Could you check a few things on this model? Use its own coordinates, in mm. Give positions to 0.01 mm unless a question says otherwise; leave off trailing zeros. Order: outer loops, then holes, each group sorted by start corner. A loop starts at its lowest first (then second) coordinate and runs counter-clockwise, first axis right, second up.
from build123d import *

# Parameters (mm, degrees)
SKETCH_R        = 50
PAD_DEPTH       = 32
SKETCH001_R     = 48
POCKET_DEPTH    = 30
SKETCH002_R     = 4
PAD001_DEPTH    = 30
SKETCH005_W     = 9.3
SKETCH005_H     = 11.3
POCKET001_DEPTH = 10
SKETCH006_W     = 6
SKETCH006_H     = 9
PAD004_DEPTH    = 10
POCKET002_DEPTH = 8
SKETCH009_R     = 5
PAD006_DEPTH    = 4
SKETCH011_W     = 0.5
SKETCH011_H     = 9.3
PAD007_DEPTH    = 0.5
SKETCH012_R     = 5
PAD008_DEPTH    = 3
POCKET004_DEPTH = 2
SKETCH014_R     = 1.5
POCKET005_DEPTH = 4
POCKET006_DEPTH = 2
SKETCH015_R     = 1.5
POCKET007_DEPTH = 5
SKETCH016_R     = 2
POCKET008_DEPTH = 5.8


with BuildPart() as part:
    # Sketch → Pad (new body)
    with BuildSketch(Plane.XY):
        Circle(SKETCH_R)
    extrude(amount=PAD_DEPTH)

    # Sketch001 (on DatumPlane) → Pocket (cut)
    with BuildSketch(Plane.XY.offset(32)):
        Circle(SKETCH001_R)
    extrude(amount=-POCKET_DEPTH, mode=Mode.SUBTRACT)

    # Sketch002 (on DatumPlane) → Pad001 (join)
    with BuildSketch(Plane.XY.offset(32)):
        with Locations((-36.373067, 21)):
            Circle(SKETCH002_R)
        with Locations((0, -42)):
            Circle(SKETCH002_R)
        with Locations((36.373067, 21)):
            Circle(SKETCH002_R)
    extrude(amount=-PAD001_DEPTH)

    # Sketch005 (on DatumPlane) → Pocket001 (cut)
    with BuildSketch(Plane.YZ.offset(50)):
        with Locations((0, 7.65)):
            Rectangle(SKETCH005_W, SKETCH005_H)
    extrude(amount=-POCKET001_DEPTH, mode=Mode.SUBTRACT)

    # Sketch006 (on DatumPlane) → Pad004 (join)
    with BuildSketch(Plane.XY.offset(2)):
        with Locations((40, 0)):
            Rectangle(SKETCH006_W, SKETCH006_H)
    extrude(amount=PAD004_DEPTH)

    # Sketch007 (on Face14 of Pad004) → Pocket002 (cut)
    with BuildSketch(Plane(origin=(37, 0, 0), x_dir=(0, -1, 0), z_dir=(-1, 0, 0))):
        with BuildLine():
            ThreePointArc((-3.99875, 6.6), (0, 2.7), (3.99875, 6.6))
            Line((5.575286, 6.6), (3.99875, 6.6))
            Line((5.575286, 15.969053), (5.575286, 6.6))
            Line((-6.906295, 15.969053), (5.575286, 15.969053))
            Line((-6.906295, 6.6), (-6.906295, 15.969053))
            Line((-3.99875, 6.6), (-6.906295, 6.6))
        make_face()
    extrude(amount=-POCKET002_DEPTH, mode=Mode.SUBTRACT)

    # Sketch009 (on DatumPlane) → Pad006 (join)
    with BuildSketch(Plane.XY.offset(2)):
        with Locations((-22.75, 32.75)):
            Circle(SKETCH009_R)
        with Locations((22.75, 32.75)):
            Circle(SKETCH009_R)
        with Locations((22.75, -32.75)):
            Circle(SKETCH009_R)
        with Locations((-22.75, -32.75)):
            Circle(SKETCH009_R)
    extrude(amount=PAD006_DEPTH)

    # Sketch011 (on DatumPlane) → Pad007 (join)
    with BuildSketch(Plane.XY.offset(2)):
        with Locations((49.533305, 0)):
            Rectangle(SKETCH011_W, SKETCH011_H)
    extrude(amount=PAD007_DEPTH)

    # Sketch012 (on DatumPlane) → Pad008 (join)
    with BuildSketch(Plane.XY.offset(2)):
        with Locations((37.35, -11.5)):
            Circle(SKETCH012_R)
    pad008 = extrude(amount=PAD008_DEPTH)

    # Sketch013 (on Face33 of Pad008) → Pocket004 (cut)
    with BuildSketch(Plane.XY.offset(5)):
        Polygon((39.95, -13.001111), (39.95, -9.998889), (37.35, -8.497779), (34.75, -9.998889), (34.75, -13.001111), (37.35, -14.502221), align=None)
    pocket004 = extrude(amount=-POCKET004_DEPTH, mode=Mode.SUBTRACT)

    # Sketch014 (on Face33 of Pocket004) → Pocket005 (cut)
    with BuildSketch(Plane.XY.offset(5)):
        with Locations((37.35, -11.5)):
            Circle(SKETCH014_R)
    pocket005 = extrude(amount=-POCKET005_DEPTH, mode=Mode.SUBTRACT)

    # Sketch010 (on DatumPlane) → Pocket006 (cut)
    with BuildSketch(Plane.XY.offset(6)):
        Polygon((-20.15, 31.248889), (-20.15, 34.251111), (-22.75, 35.752221), (-25.35, 34.251111), (-25.35, 31.248889), (-22.75, 29.747779), align=None)
        Polygon((25.35, -34.251111), (25.35, -31.248889), (22.75, -29.747779), (20.15, -31.248889), (20.15, -34.251111), (22.75, -35.752221), align=None)
        Polygon((22.75, 35.752221), (20.15, 34.251111), (20.15, 31.248889), (22.75, 29.747779), (25.35, 31.248889), (25.35, 34.251111), align=None)
        Polygon((-20.15, -31.248889), (-22.75, -29.747779), (-25.35, -31.248889), (-25.35, -34.251111), (-22.75, -35.752221), (-20.15, -34.251111), align=None)
    extrude(amount=-POCKET006_DEPTH, mode=Mode.SUBTRACT)

    # Sketch015 (on DatumPlane) → Pocket007 (cut)
    with BuildSketch(Plane.XY.offset(6)):
        with Locations((-22.75, 32.75)):
            Circle(SKETCH015_R)
        with Locations((22.75, 32.75)):
            Circle(SKETCH015_R)
        with Locations((22.7, -32.75)):
            Circle(SKETCH015_R)
        with Locations((-22.75, -32.75)):
            Circle(SKETCH015_R)
    extrude(amount=-POCKET007_DEPTH, mode=Mode.SUBTRACT)

    # Sketch016 (on DatumPlane) → Pocket008 (cut)
    with BuildSketch(Plane.XY.offset(32)):
        with Locations((-36.373067, 21)):
            Circle(SKETCH016_R)
        with Locations((36.373067, 21)):
            Circle(SKETCH016_R)
        with Locations((0, -42)):
            Circle(SKETCH016_R)
    extrude(amount=-POCKET008_DEPTH, mode=Mode.SUBTRACT)

    # Mirrored: Pad008, Pocket004, Pocket005 across Sketch012 H_Axis
    add(pad008.mirror(Plane(origin=(0, 0, 2), x_dir=(0, 0, 1), z_dir=(0, 1, 0))))
    add(pocket004.mirror(Plane(origin=(0, 0, 2), x_dir=(0, 0, 1), z_dir=(0, 1, 0))), mode=Mode.SUBTRACT)
    add(pocket005.mirror(Plane(origin=(0, 0, 2), x_dir=(0, 0, 1), z_dir=(0, 1, 0))), mode=Mode.SUBTRACT)


solid = part.part
Item 1: Imagine slicing it at A-A on z = 29. List the corners of the cut face in (x, y) for me, then the cut area to 3 significant figures.
Findings:
outline: circle Ø100 at (0, 0); circle Ø8 at (-36.37, 21); circle Ø8 at (0, -42); circle Ø8 at (36.37, 21); hole circle Ø96 at (0, 0); hole circle Ø4 at (-36.37, 21); hole circle Ø4 at (0, -42); hole circle Ø4 at (36.37, 21)
area: 729 mm2
Item 2: Imagine slicing it at C-C on y = 0. List the corners of the cut face in (x, z) for me.
Findings:
outline: (-50, 0) - (50, 0) - (50, 2) - (49.78, 2) - (49.78, 2.5) - (49.28, 2.5) - (49.28, 2) - (43, 2) - (43, 2.7) - (37, 2.7) - (37, 2) - (-48, 2) - (-48, 32) - (-50, 32) - close; (48, 13.3) - (50, 13.3) - (50, 32) - (48, 32) - close
Item 3: For pin 1 (1.6 mm diameter, centred on y = 33, z = 5.5, fed in from +X); pin 2 (8 mm diameter, centred on y = -38, z = 4.5, fed in from +X); pin 3 (8 mm diameter, centred on x = 21, y = 34, fed in from +Z), each with a flat end and sliding along its axis, tell me the tip position at first contact or that it passes through.
Findings:
pin 1: stops at x = 38.25
pin 2: stops at x = 36.66
pin 3: stops at z = 6
Item 4: Imagine slicing it at B-B on z = 10.5. List the corners of the cut face in (x, y) for me, then the cut area to 3 significant figures.
Findings:
outline: circle Ø8 at (-36.37, 21); circle Ø8 at (0, -42); circle Ø8 at (36.37, 21); (47.77, -4.65) arc R48 cw (long way) to (47.77, 4.65) - (49.78, 4.65) arc R50 ccw (long way) to (49.78, -4.65) - close
area: 748 mm2
Item 5: Please list where these lines run through material, in increasing order: line 1 along Y through (x, z) = (0, 19); line 2 along Z through (x, y) = (2, -31); line 3 along Y through (x, z) = (-23, 18).
Findings:
line 1: y = -50 to -48, -46 to -38, 48 to 50
line 2: z = 0 to 2
line 3: y = -44.4 to -42.13, 42.13 to 44.4
Item 6: We'd pull the mould along X, two halves only. Please class faces 1 (the cylindrical face through (-0.521, -38.034, 17.21)), 2 (the flat face through (35, 23, 32)): +X half, -X half, draft (parallel to the pull), parting line (faces both ways), or undercut.
Findings:
face 1: undercut
face 2: draft
Item 7: Imagine slicing it at D-D on x = 0. List the corners of the cut face in (y, z) for me, then the cut area to 3 significant figures.
Findings:
outline: (-50, 0) - (50, 0) - (50, 32) - (48, 32) - (48, 2) - (-38, 2) - (-38, 32) - (-40, 32) - (-40, 26.2) - (-44, 26.2) - (-44, 32) - (-46, 32) - (-46, 2) - (-48, 2) - (-48, 32) - (-50, 32) - close
area: 537 mm2
